```python
from build123d import *

# Parameters (mm, degrees)
F0_W           = 100
F0_H           = 50
F0_W_2         = 96
F0_H_2         = 46
F1_DEPTH       = 65
F2_W           = 100
F2_H           = 8.5998633876
F3_DEPTH       = 62.6
F4_W           = 100
F4_H           = 50
F5_DEPTH       = 3
F6_W           = 96
F6_H           = 53.983375689
F7_DEPTH       = 80.8
F8_W           = 100
F8_H           = 100
F9_DEPTH       = 5
F10_W          = 178.9870522916
F10_H          = 171.902321279
F11_DEPTH      = 2
F12_W          = 20
F12_H          = 10
F13_DEPTH      = 25
F14_R          = 2.2
F15_DEPTH      = 3
F16_R          = 5
F17_R          = 15
F18_R          = 1.5
F19_DEPTH      = 25
F20_W          = 18.0335491896
F20_H          = 117.1614909545
F21_DEPTH      = 124.6
F21_DEPTH_BACK = 25
F23_DEPTH      = 57
F24_R          = 2
F25_DEPTH      = 57
F27_DEPTH      = 3
F29_DEPTH      = 3
F30_R          = 3


with BuildPart() as f1:
    # F0 (on Front) → F1 (new body)
    with BuildSketch(Plane.XZ):
        with Locations((50, 25)):
            Rectangle(F0_W, F0_H)
        with Locations((50, 25)):
            Rectangle(F0_W_2, F0_H_2, mode=Mode.SUBTRACT)
    extrude(amount=F1_DEPTH)

    # F2 (on face) → F3 (cut)
    with BuildSketch(Plane.XZ.offset(65)):
        with Locations((50, -4.2999316938)):
            Rectangle(F2_W, F2_H)
    extrude(amount=-F3_DEPTH, mode=Mode.SUBTRACT)

    # F4 (on face) → F5 (join)
    with BuildSketch(Plane(origin=(0, 0, 0), x_dir=(-1, 0, 0), z_dir=(0, 1, 0))):
        with Locations((-50, 25)):
            Rectangle(F4_W, F4_H)
    extrude(amount=-F5_DEPTH)

    # F6 (on face) → F7 (cut)
    with BuildSketch(Plane.XZ.offset(3)):
        with Locations((50, 28.9916878445)):
            Rectangle(F6_W, F6_H)
    extrude(amount=F7_DEPTH, mode=Mode.SUBTRACT)

    # F8 (on face) → F9 (join)
    with BuildSketch(Plane.XZ.offset(65)):
        with Locations((50, 50)):
            Rectangle(F8_W, F8_H)
    extrude(amount=-F9_DEPTH)

    # F10 (on face) → F11 (cut)
    with BuildSketch(Plane.XZ.offset(65)):
        with Locations((42.4427408725, 49.3266619742)):
            Rectangle(F10_W, F10_H)
    extrude(amount=-F11_DEPTH, mode=Mode.SUBTRACT)

    # F12 (on face) → F13 (cut)
    with BuildSketch(Plane(origin=(0, 0, 0), x_dir=(1, 0, 0), z_dir=(0, 0, -1))):
        with Locations((50, 31.5)):
            Rectangle(F12_W, F12_H)
    extrude(amount=-F13_DEPTH, mode=Mode.SUBTRACT)

    # F14 (on face) → F15 (join)
    with BuildSketch(Plane.XZ.offset(63)):
        with BuildLine():
            Line((106, 60.561312139), (105.3350197713, 60.561312139))
            ThreePointArc((105.3350197713, 60.561312139), (105.6675098856, 60.5502449231), (106, 60.561312139))
        make_face()
        with BuildLine():
            Line((100, 60.561312139), (105.3350197713, 60.561312139))
            Line((105.3350197713, 60.561312139), (106, 60.561312139))
            ThreePointArc((106, 60.561312139), (110.6649022052, 65.7117070069), (105.6772652089, 70.5502354065))
            Line((105.6772652089, 70.5502354065), (100, 70.561312139))
            Line((100, 70.561312139), (100, 60.561312139))
        make_face()
        with Locations((105.6675098856, 65.5502449231)):
            Circle(F14_R, mode=Mode.SUBTRACT)
        with BuildLine():
            Line((-5.3350197713, 60.561312139), (0, 60.561312139))
            Line((0, 60.561312139), (0, 70.561312139))
            Line((0, 70.561312139), (-5.6772652089, 70.5502354065))
            ThreePointArc((-5.6772652089, 70.5502354065), (-10.6649022052, 65.7117070069), (-6, 60.561312139))
            Line((-6, 60.561312139), (-5.3350197713, 60.561312139))
        make_face()
        with Locations((-5.6675098856, 65.5502449231)):
            Circle(F14_R, mode=Mode.SUBTRACT)
        with BuildLine():
            ThreePointArc((-6, 60.561312139), (-5.6675098856, 60.5502449231), (-5.3350197713, 60.561312139))
            Line((-5.3350197713, 60.561312139), (-6, 60.561312139))
        make_face()
    extrude(amount=-F15_DEPTH)

    # F16
    f16_edges = [f1.edges().sort_by_distance(p)[0] for p in [
        (100, -61.5, 60.561312),
        (100, -61.5, 70.561312),
        (0, -61.5, 60.561312),
        (0, -61.5, 70.561312),
    ]]
    fillet(f16_edges, radius=F16_R)

    # F17
    f17_edges = [f1.edges().sort_by_distance(p)[0] for p in [
        (98, -31.5, 2),
        (2, -31.5, 2),
        (100, -31.5, 0),
        (0, -31.5, 0),
    ]]
    fillet(f17_edges, radius=F17_R)

    # F18 (on face) → F19 (cut)
    with BuildSketch(Plane.XZ.offset(63)):
        with Locations((85, 15)):
            Circle(F18_R)
        with Locations((85, 23)):
            Circle(F18_R)
        with Locations((85, 31)):
            Circle(F18_R)
        with Locations((85, 39)):
            Circle(F18_R)
        with Locations((85, 47)):
            Circle(F18_R)
        with Locations((77, 15)):
            Circle(F18_R)
        with Locations((77, 23)):
            Circle(F18_R)
        with Locations((77, 31)):
            Circle(F18_R)
        with Locations((77, 39)):
            Circle(F18_R)
        with Locations((77, 47)):
            Circle(F18_R)
        with Locations((69, 15)):
            Circle(F18_R)
        with Locations((69, 23)):
            Circle(F18_R)
        with Locations((69, 31)):
            Circle(F18_R)
        with Locations((69, 39)):
            Circle(F18_R)
        with Locations((69, 47)):
            Circle(F18_R)
        with Locations((61, 15)):
            Circle(F18_R)
        with Locations((61, 23)):
            Circle(F18_R)
        with Locations((61, 31)):
            Circle(F18_R)
        with Locations((61, 39)):
            Circle(F18_R)
        with Locations((61, 47)):
            Circle(F18_R)
        with Locations((53, 15)):
            Circle(F18_R)
        with Locations((53, 23)):
            Circle(F18_R)
        with Locations((53, 31)):
            Circle(F18_R)
        with Locations((53, 39)):
            Circle(F18_R)
        with Locations((53, 47)):
            Circle(F18_R)
        with Locations((45, 15)):
            Circle(F18_R)
        with Locations((45, 23)):
            Circle(F18_R)
        with Locations((45, 31)):
            Circle(F18_R)
        with Locations((45, 39)):
            Circle(F18_R)
        with Locations((45, 47)):
            Circle(F18_R)
        with Locations((37, 15)):
            Circle(F18_R)
        with Locations((37, 23)):
            Circle(F18_R)
        with Locations((37, 31)):
            Circle(F18_R)
        with Locations((37, 39)):
            Circle(F18_R)
        with Locations((37, 47)):
            Circle(F18_R)
        with Locations((29, 15)):
            Circle(F18_R)
        with Locations((29, 23)):
            Circle(F18_R)
        with Locations((29, 31)):
            Circle(F18_R)
        with Locations((29, 39)):
            Circle(F18_R)
        with Locations((29, 47)):
            Circle(F18_R)
        with Locations((21, 15)):
            Circle(F18_R)
        with Locations((21, 23)):
            Circle(F18_R)
        with Locations((21, 31)):
            Circle(F18_R)
        with Locations((21, 39)):
            Circle(F18_R)
        with Locations((21, 47)):
            Circle(F18_R)
        with Locations((13, 15)):
            Circle(F18_R)
        with Locations((13, 23)):
            Circle(F18_R)
        with Locations((13, 31)):
            Circle(F18_R)
        with Locations((13, 39)):
            Circle(F18_R)
        with Locations((13, 47)):
            Circle(F18_R)
    extrude(amount=-F19_DEPTH, mode=Mode.SUBTRACT)

    # F20 (on face) → F21 (cut, two sides)
    with BuildSketch(Plane(origin=(0, 0, 0), x_dir=(0, -1, 0), z_dir=(-1, 0, 0))) as f21_sk:
        with Locations((69.0167745948, 41.4192545228)):
            Rectangle(F20_W, F20_H)
    extrude(amount=-F21_DEPTH, mode=Mode.SUBTRACT)
    extrude(f21_sk.sketch, amount=F21_DEPTH_BACK, mode=Mode.SUBTRACT)

    # F22 (on face) → F23 (join, through all)
    with BuildSketch(Plane.XZ.offset(3)):
        Polygon((88.93782569, 11.9127326198), (88.93782569, 3.2253048645), (97.1109783715, 6.1686190363), (97.1109783715, 11.9127326198), align=None)
        Polygon((2.8890216285, 11.9127326198), (2.8890216285, 6.1686190363), (11.06217431, 3.2253048645), (11.06217431, 11.9127326198), align=None)
    extrude(amount=F23_DEPTH)

    # F24 (on face) → F25 (cut, through all)
    with BuildSketch(Plane.XZ.offset(60)):
        with Locations((92.6101825469, 8.5401255637)):
            Circle(F24_R)
        with Locations((7.32162036, 8.5401255637)):
            Circle(F24_R)
    extrude(amount=-F25_DEPTH, mode=Mode.SUBTRACT)

    # F26 (on face) → F27 (join)
    with BuildSketch(Plane(origin=(0, 0, 0), x_dir=(-1, 0, 0), z_dir=(0, 1, 0))):
        with BuildLine():
            ThreePointArc((-100, 15), (-95.6066017178, 4.3933982822), (-85, 0))
            Line((-85, 0), (-15, 0))
            ThreePointArc((-15, 0), (-4.3933982822, 4.3933982822), (0, 15))
            Line((0, 15), (0, 50))
            Line((0, 50), (-100, 50))
            Line((-100, 50), (-100, 15))
        make_face()
    extrude(amount=F27_DEPTH)

    # F28 (on face) → F29 (cut)
    with BuildSketch(Plane.XZ.offset(3)):
        with BuildLine():
            ThreePointArc((2, 17), (2.2239268482, 14.4178183229), (2.8890216285, 11.9127326198))
            Line((2.8890216285, 11.9127326198), (11.06217431, 11.9127326198))
            Line((11.06217431, 11.9127326198), (11.06217431, 3.2253048645))
            ThreePointArc((11.06217431, 3.2253048645), (13.9685339382, 2.3095196295), (17, 2))
            Line((17, 2), (83, 2))
            ThreePointArc((83, 2), (86.0314660618, 2.3095196295), (88.93782569, 3.2253048645))
            Line((88.93782569, 3.2253048645), (88.93782569, 11.9127326198))
            Line((88.93782569, 11.9127326198), (97.1109783715, 11.9127326198))
            ThreePointArc((97.1109783715, 11.9127326198), (97.7760731518, 14.4178183229), (98, 17))
            Line((98, 17), (98, 50))
            Line((98, 50), (2, 50))
            Line((2, 50), (2, 17))
        make_face()
    extrude(amount=-F29_DEPTH, mode=Mode.SUBTRACT)

    # F30
    f30_edges = [f1.edges().sort_by_distance(p)[0] for p in [
        (88.937826, -30, 11.912733),
        (11.062174, -30, 11.912733),
    ]]
    fillet(f30_edges, radius=F30_R)


solid = f1.part
```
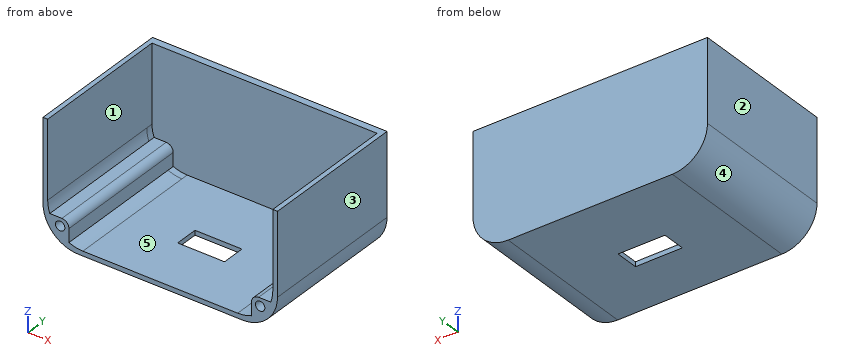
Geometry: final body of the model. Coordinates: model frame, mm. Face numbers are marked on the shaded views. A direction names the side the tool comes from. Round coordinates to 2 decimals unless told otherwise and drop trailing zeros. Order: outer loops, then holes, each group sorted by start corner. A loop starts at its lowest first (then second) coordinate and runs counter-clockwise, first axis right, second up. Notation, with made-up numbers: (1, 69.25) -> (26, 69.25) arc R14 cw to (26, 78.25) -> close; hole circle Ø5 at (73.5, 78.5). An arc over 180 degrees is marked (long way). Use one line per item in the form item = value. Start each with the question number.
1. Cut plane C-C (z = 47). Return the cut outline in (x, y), then the cut area to 3 significant figures.
2. Line query: probe 1 along X at (y, z) = (-30, 39.5); probe 2 along Y at (x, z) = (35, 21); probe 3 along Z at (x, y) = (82.5, -7). Output: solid intervals per line, ascending.
3. Cut plane B-B (y = -29.5). Return the cut outline in (x, z).
4. Pin query (flat end, axial travel): pin 1 Ø4.5 at (y, z) = (-23.5, 5) entering from -X; pin 2 Ø2 at (x, y) = (29, -3.5) entering from +Z; pin 3 Ø0.6 at (y, z) = (-30.5, 1) entering from +X. Return the tip coordinate at first contact, or that it passes through.
5. Reachability of the marked faces 4 and 5 from +Z, -Z, +X, -X, +Y, -Y: full face, straight path, thin tool, end or side. Return the list, or none.
6. Cut plane A-A (x = 48). Return the cut outline in (y, z), then the cut area to 3 significant figures.
7. Cut plane D-D (x = 71). Return the cut outline in (y, z).
8. Draft query along X for the marked faces 1, 2 and 3. Return one class per face: pulls with the +X half, pulls with the -X half, needs draft (parallel to the pull), parting line crosses it, or undercut.
Solution:
q1.outline = (0, -60) -> (2, -60) -> (2, 0) -> (98, 0) -> (98, -60) -> (100, -60) -> (100, 3) -> (0, 3) -> close
q1.area = 540 mm^2
q2.probe_1 = 0 to 2, 98 to 100
q2.probe_2 = 0 to 3
q2.probe_3 = 0 to 2
q3.outline = (0, 15) arc R15 ccw to (15, 0) -> (40, 0) -> (40, 2) -> (17, 2) arc R15 cw to (11.06, 3.23) -> (11.06, 8.91) arc R3 ccw to (8.06, 11.91) -> (2.89, 11.91) arc R15 cw to (2, 17) -> (2, 50) -> (0, 50) -> close; (60, 0) -> (85, 0) arc R15 ccw to (100, 15) -> (100, 50) -> (98, 50) -> (98, 17) arc R15 cw to (97.11, 11.91) -> (91.94, 11.91) arc R3 ccw to (88.94, 8.91) -> (88.94, 3.23) arc R15 cw to (83, 2) -> (60, 2) -> close; hole circle Ø4 at (7.32, 8.54); hole circle Ø4 at (92.61, 8.54)
q4.pin_1 = 2.16
q4.pin_2 = 2
q4.pin_3 = 91.11
q5.face_4 = -Z, -X, +Y, -Y
q5.face_5 = +Z, -Y
q6.outline = (-60, 0) -> (-36.5, 0) -> (-36.5, 2) -> (-60, 2) -> close; (-26.5, 0) -> (3, 0) -> (3, 50) -> (0, 50) -> (0, 2) -> (-26.5, 2) -> close
q6.area = 250 mm^2
q7.outline = (-60, 0) -> (3, 0) -> (3, 50) -> (0, 50) -> (0, 2) -> (-60, 2) -> close
q8.face_1 = undercut
q8.face_2 = pulls with the -X half
q8.face_3 = pulls with the +X half
